from build123d import *

# Parameters (mm, degrees)
BOSS_EXTRUDE1_DEPTH = 2.5
CHAMFER1_SIZE       = 1.25
SKETCH2_R           = 1.35
CUT_EXTRUDE1_DEPTH  = 62.140801434
BOSS_EXTRUDE2_DEPTH = 1.5
CHAMFER2_SIZE       = 1.5
CHAMFER2_SIZE_2     = 1.636962752


with BuildPart() as part:
    # Sketch1 → Boss-Extrude1 (new body)
    with BuildSketch(Plane.XY):
        with BuildLine():
            Line((49.586181166, 25), (-49.586181166, 25))
            ThreePointArc((-49.586181166, 25), (-52.267168909, 22.996486369), (-53.890165841, 20.069432712))
            ThreePointArc((-53.890165841, 20.069432712), (-55.74, 0), (-53.890165841, -20.069432712))
            ThreePointArc((-53.890165841, -20.069432712), (-51.813555608, -23.178667596), (-48.548222563, -25))
            Line((-48.548222563, -25), (48.548222563, -25))
            ThreePointArc((48.548222563, -25), (51.813555608, -23.178667596), (53.890165841, -20.069432712))
            ThreePointArc((53.890165841, -20.069432712), (55.74, 0), (53.890165841, 20.069432712))
            ThreePointArc((53.890165841, 20.069432712), (52.267168909, 22.996486369), (49.586181166, 25))
        make_face()
        with BuildLine():
            Line((-40.665, 14.165), (40.665, 14.165))
            ThreePointArc((40.665, 14.165), (44.200533906, 12.700533906), (45.665, 9.165))
            Line((45.665, 9.165), (45.665, -9.165))
            ThreePointArc((45.665, -9.165), (44.200533906, -12.700533906), (40.665, -14.165))
            Line((40.665, -14.165), (-40.665, -14.165))
            ThreePointArc((-40.665, -14.165), (-44.200533906, -12.700533906), (-45.665, -9.165))
            Line((-45.665, -9.165), (-45.665, 9.165))
            ThreePointArc((-45.665, 9.165), (-44.200533906, 12.700533906), (-40.665, 14.165))
        make_face(mode=Mode.SUBTRACT)
    extrude(amount=BOSS_EXTRUDE1_DEPTH)

    # Chamfer1
    chamfer1_edges = [part.edges().sort_by_distance(p)[0] for p in [
        (0, 25, 2.5),
    ]]
    chamfer(chamfer1_edges, length=CHAMFER1_SIZE)
    chamfer1_2_edges = [part.edges().sort_by_distance(p)[0] for p in [
        (-55.74, 0, 2.5),
    ]]
    chamfer(chamfer1_2_edges, length=CHAMFER1_SIZE)
    chamfer1_3_edges = [part.edges().sort_by_distance(p)[0] for p in [
        (0, -25, 2.5),
    ]]
    chamfer(chamfer1_3_edges, length=CHAMFER1_SIZE)
    chamfer1_4_edges = [part.edges().sort_by_distance(p)[0] for p in [
        (55.74, 0, 2.5),
    ]]
    chamfer(chamfer1_4_edges, length=CHAMFER1_SIZE)
    chamfer1_5_edges = [part.edges().sort_by_distance(p)[0] for p in [
        (51.737177521, 23.54787863, 2.5),
    ]]
    chamfer(chamfer1_5_edges, length=CHAMFER1_SIZE)
    chamfer1_6_edges = [part.edges().sort_by_distance(p)[0] for p in [
        (-51.737177521, 23.54787863, 2.5),
    ]]
    chamfer(chamfer1_6_edges, length=CHAMFER1_SIZE)
    chamfer1_7_edges = [part.edges().sort_by_distance(p)[0] for p in [
        (-51.5906008, -23.376861633, 2.5),
    ]]
    chamfer(chamfer1_7_edges, length=CHAMFER1_SIZE)
    chamfer1_8_edges = [part.edges().sort_by_distance(p)[0] for p in [
        (51.5906008, -23.376861633, 2.5),
    ]]
    chamfer(chamfer1_8_edges, length=CHAMFER1_SIZE)

    # Sketch2 → Cut-Extrude1 (cut, through all)
    with BuildSketch(Plane.XY.offset(2.5)):
        with Locations((-48.007044757, -17.939600751)):
            Circle(SKETCH2_R)
        with Locations((-49.574960594, 18.555541297)):
            Circle(SKETCH2_R)
        with Locations((48.233851408, 17.848510138)):
            Circle(SKETCH2_R)
        with Locations((48.007044757, -17.939600751)):
            Circle(SKETCH2_R)
    extrude(amount=-CUT_EXTRUDE1_DEPTH, mode=Mode.SUBTRACT)

    # Sketch3 → Boss-Extrude2 (add)
    with BuildSketch(Plane.XY.offset(2.5)):
        with BuildLine():
            Line((49.165, -9.165), (49.165, 9.165))
            ThreePointArc((49.165, 9.165), (46.67540764, 15.17540764), (40.665, 17.665))
            Line((40.665, 17.665), (-40.665, 17.665))
            ThreePointArc((-40.665, 17.665), (-46.67540764, 15.17540764), (-49.165, 9.165))
            Line((-49.165, 9.165), (-49.165, -9.165))
            ThreePointArc((-49.165, -9.165), (-46.67540764, -15.17540764), (-40.665, -17.665))
            Line((-40.665, -17.665), (40.665, -17.665))
            ThreePointArc((40.665, -17.665), (46.67540764, -15.17540764), (49.165, -9.165))
        make_face()
        with BuildLine():
            Line((44.165, -9.165), (44.165, 9.165))
            ThreePointArc((44.165, 9.165), (43.139873734, 11.639873734), (40.665, 12.665))
            Line((40.665, 12.665), (-40.665, 12.665))
            ThreePointArc((-40.665, 12.665), (-43.139873734, 11.639873734), (-44.165, 9.165))
            Line((-44.165, 9.165), (-44.165, -9.165))
            ThreePointArc((-44.165, -9.165), (-43.139873734, -11.639873734), (-40.665, -12.665))
            Line((-40.665, -12.665), (40.665, -12.665))
            ThreePointArc((40.665, -12.665), (43.139873734, -11.639873734), (44.165, -9.165))
        make_face(mode=Mode.SUBTRACT)
    extrude(amount=BOSS_EXTRUDE2_DEPTH)

    # Chamfer2
    # the kernel refuses this chamfer: 1.636962752, 1.5 mm, written as the material it takes off along each edge
    with BuildSketch(Plane(origin=(-40.665, 9.165, 4), x_dir=(0, 1, 0), z_dir=(1, 0, 0))) as chamfer2_piece_1:
        Polygon((3.5 + CHAMFER2_SIZE, 0), (3.5, -CHAMFER2_SIZE_2), (3.5, 0), align=None)
    revolve(axis=Axis((-40.665, 9.165, 4), (0, 0, 1)), revolution_arc=90, mode=Mode.SUBTRACT)
    with BuildSketch(Plane(origin=(-44.165, 9.165, 4), x_dir=(-0.9995117036729907, 0, 0.031246667353746753), z_dir=(0, -1, 0)), Plane(origin=(44.165, -9.165, 4), x_dir=(0.9995117036729907, 0, 0.031246667353746753), z_dir=(0, 1, 0))) as chamfer2_piece_2:
        Polygon((CHAMFER2_SIZE * 0.999511703673, CHAMFER2_SIZE * 0.0312466673537), (-CHAMFER2_SIZE_2 * 0.0312466673462, CHAMFER2_SIZE_2 * 0.999511703431), (0, 0), align=None)
    extrude(amount=18.33, mode=Mode.SUBTRACT)
    with BuildSketch(Plane(origin=(-40.665, -9.165, 4), x_dir=(-1, 0, 0), z_dir=(0, 1, 0))) as chamfer2_piece_3:
        Polygon((3.5 + CHAMFER2_SIZE, 0), (3.5, -CHAMFER2_SIZE_2), (3.5, 0), align=None)
    revolve(axis=Axis((-40.665, -9.165, 4), (0, 0, 1)), revolution_arc=90, mode=Mode.SUBTRACT)
    with BuildSketch(Plane(origin=(-40.665, -12.665, 4), x_dir=(0, -0.9995117036729907, 0.031246667353746788), z_dir=(1, 0, 0)), Plane(origin=(40.665, 12.665, 4), x_dir=(0, 0.9995117036729907, 0.031246667353746788), z_dir=(-1, 0, 0))) as chamfer2_piece_4:
        Polygon((CHAMFER2_SIZE * 0.999511703673, CHAMFER2_SIZE * 0.0312466673537), (-CHAMFER2_SIZE_2 * 0.0312466673462, CHAMFER2_SIZE_2 * 0.999511703431), (0, 0), align=None)
    extrude(amount=81.33, mode=Mode.SUBTRACT)
    with BuildSketch(Plane(origin=(40.665, -9.165, 4), x_dir=(0, -1, 0), z_dir=(-1, 0, 0))) as chamfer2_piece_5:
        Polygon((3.5 + CHAMFER2_SIZE, 0), (3.5, -CHAMFER2_SIZE_2), (3.5, 0), align=None)
    revolve(axis=Axis((40.665, -9.165, 4), (0, 0, 1)), revolution_arc=90, mode=Mode.SUBTRACT)
    with BuildSketch(Plane(origin=(40.665, 9.165, 4), x_dir=(1, 0, 0), z_dir=(0, -1, 0))) as chamfer2_piece_6:
        Polygon((3.5 + CHAMFER2_SIZE, 0), (3.5, -CHAMFER2_SIZE_2), (3.5, 0), align=None)
    revolve(axis=Axis((40.665, 9.165, 4), (0, 0, 1)), revolution_arc=90, mode=Mode.SUBTRACT)
    with BuildSketch(Plane(origin=(49.165, -9.165, 4), x_dir=(0.03124666735374564, 0, -0.9995117036729907), z_dir=(0, 1, 0))) as chamfer2_piece_7_section:
        Polygon((CHAMFER2_SIZE * 0.999511703673, CHAMFER2_SIZE * 0.0312466673537), (-CHAMFER2_SIZE_2 * 0.0312466673462, CHAMFER2_SIZE_2 * 0.999511703431), (0, 0), align=None)
    chamfer2_piece_7 = extrude(amount=18.33, mode=Mode.PRIVATE)
    chamfer2_piece_7 = split(chamfer2_piece_7, bisect_by=Plane(origin=(48.622856571, 0, 2.5), z_dir=(0, 0, 1)), keep=Keep.TOP, mode=Mode.PRIVATE)
    add(chamfer2_piece_7, mode=Mode.SUBTRACT)
    with BuildSketch(Plane(origin=(40.665, -9.165, 4), x_dir=(0, -1, 0), z_dir=(-1, 0, 0))) as chamfer2_piece_8_section:
        Polygon((8.5, -CHAMFER2_SIZE), (8.5 - CHAMFER2_SIZE_2, 0), (8.5, 0), align=None)
    chamfer2_piece_8 = revolve(axis=Axis((40.665, -9.165, 4), (0, 0, 1)), revolution_arc=90, mode=Mode.PRIVATE)
    chamfer2_piece_8 = split(chamfer2_piece_8, bisect_by=Plane(origin=(46.09185199, -14.59185199, 2.5), z_dir=(0, 0, 1)), keep=Keep.TOP, mode=Mode.PRIVATE)
    add(chamfer2_piece_8, mode=Mode.SUBTRACT)
    with BuildSketch(Plane(origin=(-40.665, -17.665, 4), x_dir=(0, -0.03124666735374564, -0.9995117036729907), z_dir=(1, 0, 0))) as chamfer2_piece_9_section:
        Polygon((CHAMFER2_SIZE * 0.999511703673, CHAMFER2_SIZE * 0.0312466673537), (-CHAMFER2_SIZE_2 * 0.0312466673462, CHAMFER2_SIZE_2 * 0.999511703431), (0, 0), align=None)
    chamfer2_piece_9 = extrude(amount=81.33, mode=Mode.PRIVATE)
    chamfer2_piece_9 = split(chamfer2_piece_9, bisect_by=Plane(origin=(0, -17.122856571, 2.5), z_dir=(0, 0, 1)), keep=Keep.TOP, mode=Mode.PRIVATE)
    add(chamfer2_piece_9, mode=Mode.SUBTRACT)
    with BuildSketch(Plane(origin=(-40.665, -9.165, 4), x_dir=(-1, 0, 0), z_dir=(0, 1, 0))) as chamfer2_piece_10_section:
        Polygon((8.5, -CHAMFER2_SIZE), (8.5 - CHAMFER2_SIZE_2, 0), (8.5, 0), align=None)
    chamfer2_piece_10 = revolve(axis=Axis((-40.665, -9.165, 4), (0, 0, 1)), revolution_arc=90, mode=Mode.PRIVATE)
    chamfer2_piece_10 = split(chamfer2_piece_10, bisect_by=Plane(origin=(-46.09185199, -14.59185199, 2.5), z_dir=(0, 0, 1)), keep=Keep.TOP, mode=Mode.PRIVATE)
    add(chamfer2_piece_10, mode=Mode.SUBTRACT)
    with BuildSketch(Plane(origin=(-49.165, 9.165, 4), x_dir=(-0.03124666735374564, 0, -0.9995117036729907), z_dir=(0, -1, 0))) as chamfer2_piece_11_section:
        Polygon((CHAMFER2_SIZE * 0.999511703673, CHAMFER2_SIZE * 0.0312466673537), (-CHAMFER2_SIZE_2 * 0.0312466673462, CHAMFER2_SIZE_2 * 0.999511703431), (0, 0), align=None)
    chamfer2_piece_11 = extrude(amount=18.33, mode=Mode.PRIVATE)
    chamfer2_piece_11 = split(chamfer2_piece_11, bisect_by=Plane(origin=(-48.622856571, 0, 2.5), z_dir=(0, 0, 1)), keep=Keep.TOP, mode=Mode.PRIVATE)
    add(chamfer2_piece_11, mode=Mode.SUBTRACT)
    with BuildSketch(Plane(origin=(-40.665, 9.165, 4), x_dir=(0, 1, 0), z_dir=(1, 0, 0))) as chamfer2_piece_12_section:
        Polygon((8.5, -CHAMFER2_SIZE), (8.5 - CHAMFER2_SIZE_2, 0), (8.5, 0), align=None)
    chamfer2_piece_12 = revolve(axis=Axis((-40.665, 9.165, 4), (0, 0, 1)), revolution_arc=90, mode=Mode.PRIVATE)
    chamfer2_piece_12 = split(chamfer2_piece_12, bisect_by=Plane(origin=(-46.09185199, 14.59185199, 2.5), z_dir=(0, 0, 1)), keep=Keep.TOP, mode=Mode.PRIVATE)
    add(chamfer2_piece_12, mode=Mode.SUBTRACT)
    with BuildSketch(Plane(origin=(40.665, 17.665, 4), x_dir=(0, 0.03124666735374564, -0.9995117036729907), z_dir=(-1, 0, 0))) as chamfer2_piece_13_section:
        Polygon((CHAMFER2_SIZE * 0.999511703673, CHAMFER2_SIZE * 0.0312466673537), (-CHAMFER2_SIZE_2 * 0.0312466673462, CHAMFER2_SIZE_2 * 0.999511703431), (0, 0), align=None)
    chamfer2_piece_13 = extrude(amount=81.33, mode=Mode.PRIVATE)
    chamfer2_piece_13 = split(chamfer2_piece_13, bisect_by=Plane(origin=(0, 17.122856571, 2.5), z_dir=(0, 0, 1)), keep=Keep.TOP, mode=Mode.PRIVATE)
    add(chamfer2_piece_13, mode=Mode.SUBTRACT)
    with BuildSketch(Plane(origin=(40.665, 9.165, 4), x_dir=(1, 0, 0), z_dir=(0, -1, 0))) as chamfer2_piece_14_section:
        Polygon((8.5, -CHAMFER2_SIZE), (8.5 - CHAMFER2_SIZE_2, 0), (8.5, 0), align=None)
    chamfer2_piece_14 = revolve(axis=Axis((40.665, 9.165, 4), (0, 0, 1)), revolution_arc=90, mode=Mode.PRIVATE)
    chamfer2_piece_14 = split(chamfer2_piece_14, bisect_by=Plane(origin=(46.09185199, 14.59185199, 2.5), z_dir=(0, 0, 1)), keep=Keep.TOP, mode=Mode.PRIVATE)
    add(chamfer2_piece_14, mode=Mode.SUBTRACT)


solid = part.part
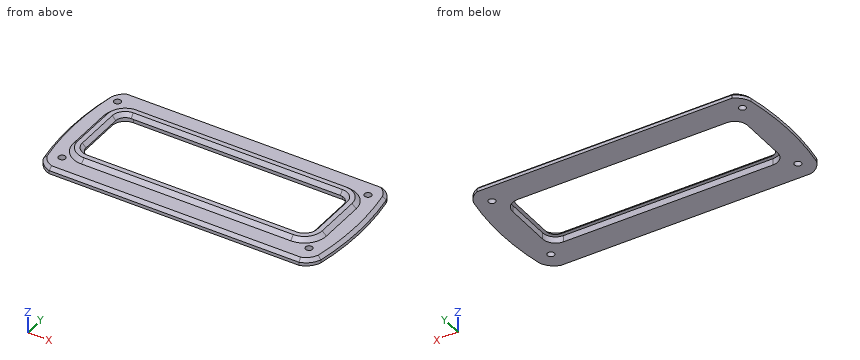
Part model, mm, in its own coordinate system. Coordinates: 2 decimals unless noted, no trailing zeros. Order: outer loops, then holes, each group sorted by start corner. A loop starts at its lowest first (then second) coordinate and runs counter-clockwise, first axis right, second up.
(1) Pin check, flat tips, straight feed: pin 1 Ø3.5 at (x, y) = (48.01, -17.94) entering from -Z; pin 2 Ø3.5 at (x, y) = (-49.57, 18.56) entering from +Z; pin 3 Ø8.5 at (x, y) = (19.5, 4.5) entering from -Z; pin 4 Ø2 at (y, z) = (7.5, 0.5) entering from -X. Stop position of each tip, or through.
Check sheet entries:
pin 1: stops at z = 0
pin 2: stops at z = 2.5
pin 3: passes through
pin 4: stops at x = -55.55
(2) Probe L1, parallel to Y at x = 35, z = 0.7 (3 decimals); L2, parallel to X at y = -6.5, z = 2.45 (3 decimals); L3, parallel to Y at x = -49, z = 2.3. List the from-to ranges inside material, lowest first.
Check sheet entries:
L1: y = -25 to -14.165, 14.165 to 25
L2: x = -54.345 to -45.665, 45.665 to 54.345
L3: y = -23.74 to -18.85, -17.02 to 17.33, 19.78 to 23.95
(3) Slice it at C-C, the plane z = 3.3. Write the cut outline in (x, y) (3 decimals).
Check sheet entries:
outline: (-48.292, -9.165) arc R7.627 ccw to (-40.665, -16.792) - (40.665, -16.792) arc R7.627 ccw to (48.292, -9.165) - (48.292, 9.165) arc R7.627 ccw to (40.665, 16.792) - (-40.665, 16.792) arc R7.627 ccw to (-48.292, 9.165) - close; hole (-45.024, -9.165) arc R4.359 ccw to (-40.665, -13.524) - (40.665, -13.524) arc R4.359 ccw to (45.024, -9.165) - (45.024, 9.165) arc R4.359 ccw to (40.665, 13.524) - (-40.665, 13.524) arc R4.359 ccw to (-45.024, 9.165) - close
